```python
from build123d import *

# Parameters (mm, degrees)
BOSS_EXTRU_1_DEPTH = 36
CHANFREIN1_SIZE    = 7
CHANFREIN2_SIZE    = 10


with BuildPart() as part:
    # Esquisse1 → Boss.-Extru.1 (new body)
    with BuildSketch(Plane(origin=(0, 0, 0), x_dir=(1, 0, 0), z_dir=(0, 1, 0))):
        Polygon((43.253574696, -35.237781767), (-13.693473115, 92.656837923), (-95.979938868, -20.608061997), align=None)
    extrude(amount=BOSS_EXTRU_1_DEPTH)

    # Chanfrein1
    chanfrein1_edges = [part.edges().sort_by_distance(p)[0] for p in [
        (-54.836705991, 36, -36.024387963),
        (-54.836705991, 0, -36.024387963),
        (-26.363182086, 36, 27.922921882),
        (14.780050791, 0, -28.709528078),
        (-26.363182086, 0, 27.922921882),
        (14.780050791, 36, -28.709528078),
    ]]
    chamfer(chanfrein1_edges, length=CHANFREIN1_SIZE)

    # Chanfrein2
    chanfrein2_edges = [part.edges().sort_by_distance(p)[0] for p in [
        (-13.693473115, 18, -92.656837923),
        (43.253574696, 18, 35.237781767),
        (-95.979938868, 18, 20.608061997),
    ]]
    chamfer(chanfrein2_edges, length=CHANFREIN2_SIZE)


solid = part.part
```
Part model, mm, in its own coordinate system. Round coordinates to 2 decimals unless told otherwise and drop trailing zeros. Write each loop counter-clockwise with the first axis right and the second up, starting at its lowest first coordinate (ties: lowest second). Pieces come first, ordered by that corner, then holes.
Item 1: Probe L1, parallel to Z at x = -82, y = 27; L2, parallel to Z at x = 19, y = 15; L3, parallel to X at y = 12, z = -70. List the from-to ranges inside material, lowest first.
Results:
L1: z = 1.37 to 22.08
L2: z = -19.23 to 32.69
L3: x = -30.15 to -3.61
Item 2: Cut at C-C, the plane y = 4.5. Give the cut face in (x, z).
Results:
outline: (-88.93, 15.15) - (-16.7, -84.26) - (-12.5, -83.82) - (37.49, 28.44) - (35.01, 31.86) - (-87.21, 19.02) - close
Item 3: Drop flat-ended pins along their axis: pin 1 Ø1.5 at (x, z) = (-66.5, 18) entering from +Y; pin 2 Ø6 at (y, z) = (10, -66.5) entering from +X; pin 3 Ø10 at (x, y) = (-60.5, 31.5) entering from +Z. Give the stop position or say it passes through.
Results:
pin 1: stops at y = 35.42
pin 2: stops at x = -0.71
pin 3: stops at z = 24.79
Item 4: Cut at B-B, the plane x = -3.5. Give the cut face in (y, z).
Results:
outline: (0, -52.55) - (7, -69.76) - (29, -69.76) - (36, -52.55) - (36, 23.29) - (29, 30.33) - (7, 30.33) - (0, 23.29) - close
Item 5: Cut at D-D, the plane y = 30.5. Give the cut face in (x, z).
Results:
outline: (-89.4, 14.1) - (-17.85, -84.39) - (-11.35, -83.7) - (38.17, 27.5) - (34.33, 32.79) - (-86.74, 20.07) - close
Item 6: Cut at A-A, the plane z = -30.5. Give the cut face in (x, y), plus the area to 3 significant figures.
Results:
outline: (-58.85, 7) - (-50.2, 0) - (6.32, 0) - (13.98, 7) - (13.98, 29) - (6.32, 36) - (-50.2, 36) - (-58.85, 29) - close
area: 2,510 mm2
